Autodesk Inventor part; units mm, degrees
ref_plane "YZ Plane" through (0, 0, 0) normal (1, 0, 0) x (0, 1, 0)
ref_plane "XZ Plane" through (0, 0, 0) normal (0, 1, 0) x (-1, 0, 0)
ref_plane "XY Plane" through (0, 0, 0) normal (0, 0, 1) x (1, 0, 0)
sketch "Sketch1" plane through (0, 0, 0) normal (0, 0, 1) x (1, 0, 0)
  line L0 (-54.464, 10.0328) -> (58.286, 10.0328)
  line L1 (58.286, 10.0328) -> (58.286, -10.415)
  line L2 (58.286, -10.415) -> (-54.464, -10.415)
  line L3 (-54.464, -10.415) -> (-54.464, 10.0328)
  line L4 (58.286, 5.794) -> (65.556, 5.794)
  line L5 (65.556, 5.794) -> (65.556, -5.8813)
  line L6 (65.556, -5.8813) -> (58.286, -5.8813)
  line L7 (58.286, -5.8813) -> (58.286, 5.794)
  point P0 (0, 0)
  dimension "d0" = 112.75
  dimension "d1" = 120.02
extrude "Extrusion1" add sketch "Sketch1" along normal blind 2
chamfer "Chamfer1" distance 4.2 angle 45 2 edges at (58.286, 10.0328, 1) (58.286, -10.415, 1)
fillet "Fillet1" radius 2 2 edges at (65.556, 5.794, 1) (65.556, -5.8813, 1)
sketch "Sketch3" plane through (-54.464, -10.415, 0) normal (-1, 0, 0) x (0, 0, 1)
  line L0 (0, 20.4479) -> (0, 0)
  line L1 (0, 17.9079) -> (13.43, 17.9079)
  line L2 (13.43, 17.9079) -> (13.43, -3.6821)
  line L3 (13.43, -3.6821) -> (0, -3.6821)
  line L4 (0, -3.6821) -> (0, 17.9079)
  line L5 (0, 20.4479) -> (2, 20.4479)
  line L6 (2, 20.4479) -> (2, 0)
  point P0 (0, 10.415)
  dimension "d14" = 2.54
  dimension "d15" = 21.59
  dimension "d16" = 11.43
extrude "Extrusion3" add sketch "Sketch3" along normal blind 1.5 contours L1 L2 L3 L4 L0
sketch "Sketch4" plane through (0, 0, 0) normal (0, 0, -1) x (-1, 0, 0)
  line L0 (55.964, -14.0972) -> (55.964, 7.4928)
  line L1 (-54.086, 10.0328) -> (54.464, 10.0328)
  line L2 (55.964, 7.4928) -> (52.024, 7.4928)
  line L3 (52.024, 7.4928) -> (52.024, 10.0328)
  line L4 (52.024, 10.0328) -> (55.964, 10.0328)
  line L5 (55.964, 10.0328) -> (55.964, 7.4928)
  point P0 (0, 0)
  point P1 (-30.556, 10.0328)
  dimension "d19" = 3.94
extrude "Extrusion4" cut sketch "Sketch4" against normal blind 20
chamfer "Chamfer3" distance 2.54 angle 45 1 edges at (-52.024, 10.0328, 1)
chamfer "Chamfer4" distance 3.68 angle 45 1 edges at (-54.464, -10.415, 1)
fillet "Fillet2" radius 3 2 edges at (-55.214, 7.4928, 13.43) (-55.214, -14.0972, 13.43)
sketch "Sketch5" plane through (-55.964, -10.415, 0) normal (-1, 0, 0) x (0, 0, 1)
  circle A0 centre (7.08, 2.0279) radius 2.21
  line L0 (0, -3.6821) -> (10.43, -3.6821)
  line L1 (9.29, 2.0279) -> (4.87, 2.0279)
  line L2 (4.87, 2.0279) -> (4.87, -3.6821)
  line L3 (4.87, -3.6821) -> (9.29, -3.6821)
  line L4 (9.29, -3.6821) -> (9.29, 2.0279)
  line L5 (2, 20.4479) -> (0, 20.4479)
  line L6 (2, 17.9079) -> (2, 20.4479)
  point P0 (0, 10.415)
  point P1 (7.08, 2.0279)
  point P2 (9.29, -3.6821)
  point P3 (4.87, 2.0279)
  dimension "d29" = 4.42
  dimension "d30" = 18.42
  dimension "d31" = 5.08
  dimension "d32" = 5.08
  dimension "d33" = 4.42
extrude "Extrusion5" cut sketch "Sketch5" against normal blind 2
fillet "Fillet3" radius 1 1 edges at (-54.464, -3.3011, 2)
fillet "Fillet4" radius 1 1 edges at (-55.964, -3.3022, 0)
sketch "Sketch13" plane through (0, 0, 0) normal (0, 0, -1) x (-1, 0, 0)
  line L0 (-1.036, 6.4328) -> (0.964, 6.4328)
  line L1 (0.964, 6.4328) -> (-0.036, 8.0328)
  line L2 (-0.036, 8.0328) -> (-1.036, 6.4328)
  line L3 (-54.086, 10.0328) -> (49.484, 10.0328)
  line L4 (54.964, 7.4928) -> (54.964, -14.0972)
  point P0 (0, 0)
  point P1 (-30.556, 10.0328)
  dimension "d84" = 2
  dimension "d85" = 1.6
  dimension "d86" = 1
  dimension "d87" = 2
  dimension "d88" = 55
extrude "Extrusion12" cut sketch "Sketch13" against normal blind 0.4
sketch "Sketch14" plane through (0, 0, 2) normal (0, 0, 1) x (1, 0, 0)
  line L0 (-54.464, -11.0972) -> (-54.464, 4.4928)
  line L1 (-50.784, -10.415) -> (54.086, -10.415)
  line L2 (54.086, 10.0328) -> (-49.484, 10.0328)
  point P0 (0, 0)
  point P1 (-41.464, -0.415)
  point P2 (41.536, -5.415)
  point P3 (41.536, 4.585)
  dimension "d91" = 13
  dimension "d92" = 10
  dimension "d93" = 96
  dimension "d94" = 96
  dimension "d95" = 15
  dimension "d96" = 5
  dimension "d97" = 5.4479
hole "Hole2" at (-41.464, -0.415, 2) at (41.536, -5.415, 2) at (41.536, 4.585, 2) direction (0, 0, -1) diameter 3 depth 5 tip angle 118 countersink diameter 7 countersink angle 90
sketch "Sketch17" plane through (-49.484, 10.0328, 0) normal (0, 1, 0) x (1, 0, 0)
  line L0 (103.57, -2) -> (0, -2)
  line L1 (5.02, -2) -> (100.04, -2)
  line L2 (100.04, -2) -> (100.04, 2)
  line L3 (100.04, 2) -> (5.02, 2)
  line L4 (5.02, 2) -> (5.02, -2)
  line L5 (-4.98, -10.43) -> (-4.98, -3)
  line L6 (115.04, -2) -> (115.04, 0)
  point P0 (49.484, 0)
  dimension "d114" = 4
  dimension "d115" = 10
  dimension "d116" = 15
extrude "Extrusion14" add sketch "Sketch17" against normal blind 1.2
chamfer "Chamfer8" distance 2 angle 45 2 edges at (-44.464, 9.4328, -2) (50.556, 9.4328, -2)
sketch "Sketch18" plane through (0, 0, 2) normal (0, 0, 1) x (1, 0, 0)
  line L0 (-2.964, 6.785) -> (12.536, 6.785)
  line L1 (12.536, 6.785) -> (12.536, -7.215)
  line L2 (12.536, -7.215) -> (-2.964, -7.215)
  line L3 (-2.964, -7.215) -> (-2.964, 6.785)
  circle A0 centre (41.536, 4.585) radius 1.5
  line L4 (-50.784, -10.415) -> (54.086, -10.415)
  point P0 (0, 0)
  dimension "d122" = 29
  dimension "d123" = 44.5
  dimension "d124" = 3.2
  dimension "d125" = 14
extrude "Extrusion15" cut sketch "Sketch18" against normal blind 2 contours L0 L1 L2 L3
sketch "Sketch20" plane through (0, 0, 2) normal (0, 0, 1) x (1, 0, 0)
  line L0 (65.556, -5.8813) -> (58.286, -5.8813)
  line L1 (58.286, -5.8813) -> (58.286, 5.794)
  line L2 (58.286, 5.794) -> (65.556, 5.794)
  line L3 (65.556, 5.794) -> (65.556, -5.8813)
  line L4 (58.286, -10.415) -> (51.286, -10.415)
  line L5 (51.286, -10.415) -> (51.286, 10.0328)
  line L6 (51.286, 10.0328) -> (58.286, 10.0328)
  line L7 (58.286, 10.0328) -> (58.286, -10.415)
  line L8 (65.556, -3.8813) -> (65.556, 3.794)
  line L9 (58.286, -5.8813) -> (63.556, -5.8813)
  line L10 (63.556, 5.794) -> (58.286, 5.794)
  line L11 (54.086, 10.0328) -> (-49.484, 10.0328)
  line L12 (-50.784, -10.415) -> (54.086, -10.415)
  line L13 (58.286, -6.215) -> (58.286, -5.8813)
  point P0 (0, 0)
  dimension "d136" = 7
extrude "Extrusion17" add sketch "Sketch20" along normal blind 2
chamfer "Chamfer11" distance 4.2 angle 45 2 edges at (58.286, -10.415, 3) (58.286, 10.0328, 3)
chamfer "Chamfer12" distance 2 angle 45 1 edges at (51.286, -0.1911, 2)
sketch "Sketch21" plane through (-50.784, -10.415, 0) normal (0, -1, 0) x (1, 0, 0)
  line L0 (116.34, 0) -> (114.34, 0)
  line L1 (116.34, 0) -> (103.34, 0)
  line L2 (103.34, 0) -> (103.34, 2)
  line L3 (103.34, 2) -> (116.34, 2)
  line L4 (116.34, 2) -> (116.34, 0)
  line L5 (114.34, 2) -> (116.34, 2)
  line L6 (104.87, 0) -> (101.34, 0)
  point P0 (50.784, 0)
  dimension "d145" = 2
extrude "Extrusion18" cut sketch "Sketch21" against normal blind 200
chamfer "Chamfer13" distance 2 angle 45 1 edges at (52.556, -0.1911, 0)
fillet "Fillet10" radius 3 2 edges at (65.556, -5.8813, 3) (65.556, 5.794, 3)
sketch "Sketch22" plane through (-50.784, -10.415, 0) normal (0, -1, 0) x (1, 0, 0)
  line L0 (101.14, 4) -> (116.34, 4)
  line L1 (116.34, 4) -> (116.34, 3.2)
  line L2 (116.34, 3.2) -> (101.14, 3.2)
  line L3 (101.14, 3.2) -> (101.14, 4)
  line L4 (102.07, 4) -> (104.87, 4)
  line L5 (116.34, 2) -> (116.34, 4)
  point P0 (50.784, 0)
  dimension "d152" = 15.2
  dimension "d153" = 0.8
extrude "Extrusion19" cut sketch "Sketch22" against normal blind 200
sketch "Sketch23" plane through (-49.484, 8.8328, 0) normal (0, -1, 0) x (1, 0, 0)
  line L0 (5.02, 0) -> (100.04, 0)
  line L1 (7.02, -2) -> (98.04, -2)
  line L2 (100.04, 0) -> (95.04, 0)
  line L3 (95.04, 0) -> (95.04, -2)
  line L4 (95.04, -2) -> (100.04, -2)
  line L5 (100.04, -2) -> (100.04, 0)
  point P0 (49.484, 0)
  dimension "d156" = 5
extrude "Extrusion20" cut sketch "Sketch23" against normal blind 10
chamfer "Chamfer14" distance 2 angle 45 1 edges at (45.556, 9.4328, -2)
sketch "Sketch24" plane through (-55.964, -10.415, 0) normal (-1, 0, 0) x (0, 0, 1)
  arc A0 (9.29, 2.0279) -> (4.87, 2.0279) centre (7.08, 2.0279) ccw
  circle A1 centre (7.08, 2.0279) radius 2.21
  line L0 (4.87, -3.6821) -> (4.87, 2.0279)
  line L1 (9.29, 2.0279) -> (9.29, -3.6821)
  line L2 (4.87, -3.6821) -> (9.29, -3.6821)
  line L3 (9.29, -3.6821) -> (9.29, -0.6821)
  line L4 (9.29, -0.6821) -> (4.87, -0.6821)
  line L5 (4.87, -0.6821) -> (4.87, -3.6821)
  point P0 (0, 10.415)
  point P1 (9.29, 2.0279)
  point P2 (4.87, 2.0279)
  dimension "d162" = 3
extrude "Extrusion21" add sketch "Sketch24" against normal blind 1.5 contours L1 L4 L0 A1 | L1 L2 L0 L4
chamfer "Chamfer15" distance 0.4 angle 45 1 edges at (-55.964, -8.3872, 4.87)
chamfer "Chamfer16" distance 2 angle 45 2 edges at (12.536, -0.215, 2) (-2.964, -0.215, 2)
sketch "Sketch26" plane through (0, 0, 0) normal (0, 0, -1) x (-1, 0, 0)
  line L0 (44.464, 8.8328) -> (-45.556, 8.8328)
  line L1 (-14.736, 8.8328) -> (-12.736, 8.8328)
  line L2 (-12.736, 8.8328) -> (-12.736, -6.715)
  line L3 (-12.736, -6.715) -> (-14.736, -6.715)
  line L4 (-14.736, -6.715) -> (-14.736, 8.8328)
  line L5 (3.164, 8.8328) -> (5.164, 8.8328)
  line L6 (5.164, 8.8328) -> (5.164, -6.715)
  line L7 (5.164, -6.715) -> (3.164, -6.715)
  line L8 (3.164, -6.715) -> (3.164, 8.8328)
  line L9 (-12.536, -7.215) -> (-12.536, 6.785)
  line L10 (2.964, 6.785) -> (2.964, -7.215)
  line L11 (2.964, -7.215) -> (-12.536, -7.215)
  point P0 (0, 0)
  dimension "d175" = 0.2
  dimension "d176" = 0.2
  dimension "d177" = 2
  dimension "d178" = 2
  dimension "d179" = 0.5
  dimension "d180" = 0.5
extrude "Extrusion23" add sketch "Sketch26" along normal blind 2
chamfer "Chamfer17" distance 2 angle 45 2 edges at (14.736, 8.8328, -1) (-5.164, 8.8328, -1)
properties part number "pcie-bracket"
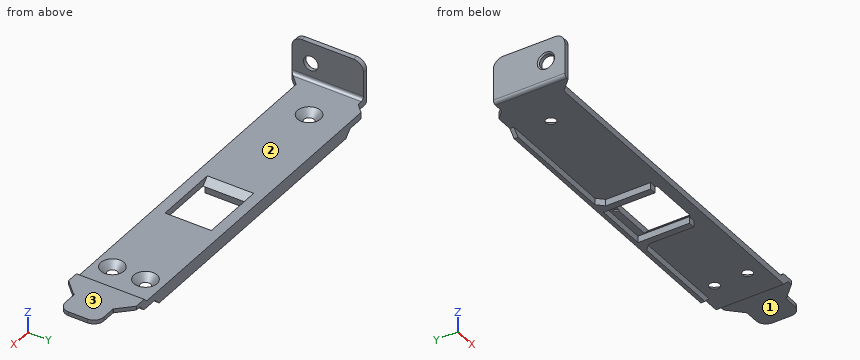
CAD build for the part. Positions are in the model's coordinates, mm. Face numbers are marked on the shaded views. A direction names the side the tool comes from. Round coordinates to 2 decimals unless told otherwise and drop trailing zeros. Order: outer loops, then holes, each group sorted by start corner. A loop starts at its lowest first (then second) coordinate and runs counter-clockwise, first axis right, second up.
Q1. Drop flat-ended pins along their axis: pin 1 (1.6 mm diameter, centred on x = 13.5, z = -1, fed in from -Y) (3 decimals); pin 2 (1.6 mm diameter, centred on y = 1, z = -0.5, fed in from -X); pin 3 (1 mm diameter, centred on x = 60, z = 2.5, fed in from +Y). Give the stop position or say it passes through.
Q2. Slice it at C-C (x = -21). Write the cut outline in (y, z) (3 decimals).
Q3. Slice it at B-B (x = 2). Write the cut outline in (y, z) (3 decimals).
Q4. Wall check: L1, parallel to Y at x = -54.75, z = 7.08; L2, parallel to X at y = 3.5, z = 0.75; L3, parallel to X at y = 5.5, z = 1.5. Give the ranges that are in metal, low to high.
Q5. Slice it at D-D (x = -46). Write the cut outline in (y, z) (3 decimals).
Q6. Which spindle directions (+Z, -Z, +X, -X, +Y, -Y) get a long thin tool onto all of the face, cutting with end or side? Do the marked faces 1, 2 and 3. Say none if no direction does.
Q7. Slice it at A-A (z = 7.08). Write the cut outline in (x, y), and give its area (3 significant figures).
Results below:
1. pin 1: stops at y = -6.715
1. pin 2: stops at x = -55.68
1. pin 3: stops at y = 5.79
2. outline: (-10.415, 0) - (8.833, 0) - (8.833, -2) - (10.033, -2) - (10.033, 2) - (-10.415, 2) - close
3. outline: (-10.415, 0) - (-7.215, 0) - (-7.215, 2) - (-10.415, 2) - close; (6.785, 0) - (8.833, 0) - (8.833, -2) - (10.033, -2) - (10.033, 2) - (6.785, 2) - close
4. L1: y = -14.1 to -10.6, -6.18 to 7.49
4. L2: x = -55.93 to -3.71, 13.29 to 39.56, 43.51 to 51.31
4. L3: x = -55.96 to -4.46, 14.04 to 38.68, 44.39 to 52.06
5. outline: (-10.415, 0) - (10.033, 0) - (10.033, 2) - (-10.415, 2) - close
6. face 1: -Z, +X, +Y, -Y
6. face 2: +Z, +Y, -Y
6. face 3: +Z, +X, +Y, -Y
7. outline: (-55.96, -14.1) - (-54.46, -14.1) - (-54.46, -10.6) - (-55.56, -10.6) - (-55.96, -11) - close; (-55.96, -5.78) - (-55.56, -6.18) - (-54.46, -6.18) - (-54.46, 7.49) - (-55.96, 7.49) - close
7. area: 25.6 mm2
